Verification items for the finished model (mm, model axes). Face numbers are marked on the shaded views. A direction names the side the tool comes from. Give positions to 0.01 mm unless a question says otherwise; leave off trailing zeros. Write each loop counter-clockwise with the first axis right and the second up, starting at its lowest first coordinate (ties: lowest second). Pieces come first, ordered by that corner, then holes. Notation, with made-up numbers: M 3.5,23.25 L 25.5,23.25 A12 ccw 25.5,43.25 Z; hole C -3,80 d5. An arc over 180 degrees is marked long. Write item = value, one per line.
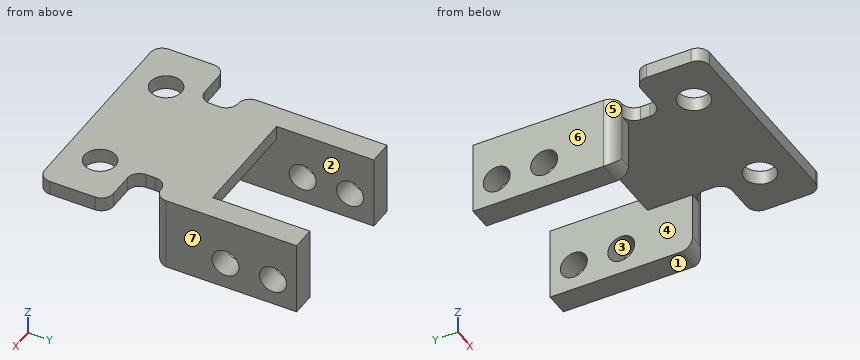
from build123d import *

# Parameters (mm, degrees)
SKETCH1_W                        = 45
SKETCH1_H                        = 14.46
BOSS_EXTRUDE1_DEPTH              = 3
F_1_4_0_2584625_DIAMETER_HOLE1_D = 6.5649475
SKETCH5_W                        = 24.2
SKETCH5_H                        = 37.04
BOSS_EXTRUDE2_DEPTH              = 3
SKETCH6_W                        = 15.5
SKETCH6_H                        = 30
BOSS_EXTRUDE3_DEPTH              = 5
BOSS_EXTRUDE4_START              = -29.2
SKETCH7_W                        = 15.5
SKETCH7_H                        = 30
BOSS_EXTRUDE4_DEPTH              = 5
SKETCH12_W                       = 24.2
SKETCH12_H                       = 20.5
CUT_EXTRUDE1_DEPTH               = 3
M5_CLEARANCE_HOLE1_D             = 5.686175
FILLET3_R                        = 2.5
FILLET4_R                        = 2.5


with BuildPart() as part:
    # Sketch1 → Boss-Extrude1 (new body)
    with BuildSketch(Plane.XY):
        with Locations((13.988651535, -1.802042724)):
            Rectangle(SKETCH1_W, SKETCH1_H)
    extrude(amount=BOSS_EXTRUDE1_DEPTH)

    # 1/4 (0.2584625) Diameter Hole1 (through all)
    with Locations(Plane(origin=(0, 0, 0), x_dir=(-1, 0, 0), z_dir=(0, 0, -1))):
        with Locations((-26.488651535, -1.532042724), (-1.488651535, -1.532042724)):
            Hole(F_1_4_0_2584625_DIAMETER_HOLE1_D / 2)

    # Sketch5 → Boss-Extrude2 (add)
    with BuildSketch(Plane(origin=(0, 0, 0), x_dir=(-1, 0, 0), z_dir=(0, 0, -1))):
        with Locations((-13.988651535, 23.947957276)):
            Rectangle(SKETCH5_W, SKETCH5_H)
    extrude(amount=-BOSS_EXTRUDE2_DEPTH)

    # Sketch6 → Boss-Extrude3 (add)
    with BuildSketch(Plane.ZY.offset(-1.888651535)):
        with Locations((-4.75, 27.467957276)):
            Rectangle(SKETCH6_W, SKETCH6_H)
    extrude(amount=BOSS_EXTRUDE3_DEPTH)

    # Sketch7 → Boss-Extrude4 (add)
    with BuildSketch(Plane.ZY.offset(3.111348465).offset(BOSS_EXTRUDE4_START)):
        with Locations((-4.75, 27.467957276)):
            Rectangle(SKETCH7_W, SKETCH7_H)
    extrude(amount=-BOSS_EXTRUDE4_DEPTH)

    # Sketch12 → Cut-Extrude1 (cut)
    with BuildSketch(Plane(origin=(0, 0, 0), x_dir=(-1, 0, 0), z_dir=(0, 0, -1))):
        with Locations((-13.988651535, 32.217957276)):
            Rectangle(SKETCH12_W, SKETCH12_H)
    extrude(amount=-CUT_EXTRUDE1_DEPTH, mode=Mode.SUBTRACT)

    # M5 Clearance Hole1 (through all)
    with Locations(Plane.ZY.offset(3.111348465)):
        with Locations((-6.85, 37.467957276), (-6.85, 27.467957276)):
            Hole(M5_CLEARANCE_HOLE1_D / 2)

    # Fillet3
    fillet3_edges = [part.edges().sort_by_distance(p)[0] for p in [
        (-8.511348465, 5.427957276, 1.5),
        (36.488651535, 5.427957276, 1.5),
        (36.488651535, -9.032042724, 1.5),
        (-8.511348465, -9.032042724, 1.5),
    ]]
    fillet(fillet3_edges, radius=FILLET3_R)

    # Fillet4
    fillet4_edges = [part.edges().sort_by_distance(p)[0] for p in [
        (1.888651535, 5.427957276, 1.5),
        (26.088651535, 5.427957276, 1.5),
        (26.088651535, 12.467957276, 1.5),
        (1.888651535, 12.467957276, 1.5),
        (31.088651535, 12.467957276, -4.75),
        (-3.111348465, 12.467957276, -4.75),
        (28.588651535, 12.467957276, -12.5),
        (-0.611348465, 12.467957276, -12.5),
    ]]
    fillet(fillet4_edges, radius=FILLET4_R - 0.0001)  # a hair under: the kernel refuses the full size


solid = part.part
1) Cross-section at B-B on z = -6.85. Record the boundary of the cut face in (x, y).
From the geometry:
outline = M -3.11,14.97 A2.5 ccw -0.61,12.47 L 1.89,12.47 L 1.89,24.62 L -3.11,24.62 Z; M -3.11,30.31 L 1.89,30.31 L 1.89,34.62 L -3.11,34.62 Z; M -3.11,40.31 L 1.89,40.31 L 1.89,42.47 L -3.11,42.47 Z; M 26.09,12.47 L 28.59,12.47 A2.5 ccw 31.09,14.97 L 31.09,24.62 L 26.09,24.62 Z; M 26.09,30.31 L 31.09,30.31 L 31.09,34.62 L 26.09,34.62 Z; M 26.09,40.31 L 31.09,40.31 L 31.09,42.47 L 26.09,42.47 Z
2) Draft check along Z on the marked faces 1, 2 and 3. Enter one of: +Z half, -Z half, draft (parallel to the pull), parting line (faces both ways), or undercut.
From the geometry:
face_1 = -Z half
face_2 = draft
face_3 = undercut
3) Cross-section at A-A on z = -2.75. Record the boundary of the cut face in (x, y).
From the geometry:
outline = M -3.11,14.97 A2.5 ccw -0.61,12.47 L 1.89,12.47 L 1.89,42.47 L -3.11,42.47 Z; M 26.09,12.47 L 28.59,12.47 A2.5 ccw 31.09,14.97 L 31.09,42.47 L 26.09,42.47 Z
4) Cross-section at C-C on y = -3. Record the boundary of the cut face in (x, z), plus the area to 3 significant figures.
From the geometry:
outline = M -8.51,0 L -1.45,0 L -1.45,3 L -8.51,3 Z; M 4.42,0 L 23.55,0 L 23.55,3 L 4.42,3 Z; M 29.42,0 L 36.49,0 L 36.49,3 L 29.42,3 Z
area = 99.8 mm^2
5) Depth check by flat-ended pin: P1, Ø9, axis at y = 37.47, z = -6.85, coming from the +X side; P2, Ø4.5, axis at y = 22.5, z = -1.5, coming from the -X side; P3, Ø1.3, axis at x = 27.5, z = -2.5, coming from the -Y side; P4, Ø4, axis at x = 9, z = -0.5, coming from the -Y side. Enter the tip coordinate at first touch or a pass-through.
From the geometry:
P1 = 31.09
P2 = -3.11
P3 = 12.47
P4 = -9.03
6) Tool access check on the marked faces 4, 5, 6 and 7. Record the directions out of +Z, -Z, +X, -X, +Y, -Y that give a thin tool (end or side, any length) a straight path to the whole face; none if there is none.
From the geometry:
face_4 = -Z, +Y
face_5 = +Z, -Z, -X
face_6 = +Z, -Z, -X, +Y
face_7 = +Z, -Z, +X, +Y
7) Material ranges on probe 1 along Y at (x, z) = (0.8, -6.85); probe 2 along X at (y, z) = (36, -9.75); probe 3 along X at (y, z) = (-2, 0.75), recorded low to high. Write a range as from..to.
From the geometry:
probe_1 = 12.47..24.62, 30.31..34.62, 40.31..42.47
probe_2 = -3.11..1.89, 26.09..31.09
probe_3 = -8.51..-1.76, 4.74..23.24, 29.74..36.49
8) Cross-section at D-D on x = 3. Record the boundary of the cut face in (y, z).
From the geometry:
outline = M -9.03,0 L -4.45,0 L -4.45,3 L -9.03,3 Z; M 1.38,0 L 21.97,0 L 21.97,3 L 1.38,3 Z
